Part model, mm, in its own coordinate system. A direction names the side the tool comes from. Give positions to 0.01 mm unless a question says otherwise; leave off trailing zeros. Write each loop counter-clockwise with the first axis right and the second up, starting at its lowest first coordinate (ties: lowest second). Pieces come first, ordered by that corner, then holes. Notation, with made-up numbers: M 26,28.25 L 52,28.25 A22 cw 52,44.25 Z; hole C -28,-16 d2. An arc over 180 degrees is marked long. Use a Markdown table: item, result.
```python
from build123d import *

# Parameters (mm, degrees)
F1_DEPTH = 4
F2_R     = 2.125
F3_DEPTH = 5.001
F4_W     = 8
F4_H     = 8
F5_DEPTH = 4
F6_R     = 2.125
F7_DEPTH = 22.001
F9_DEPTH = 4


with BuildPart() as f1:
    # F0 (on Top) → F1 (new body, symmetric)
    with BuildSketch(Plane.XY):
        with BuildLine():
            ThreePointArc((-3.2, -2.642442), (0, 4.15), (3.2, -2.642442))
            Line((3.2, -2.642442), (3.2, -17.642442))
            Line((3.2, -17.642442), (7, -17.642442))
            Line((7, -17.642442), (7, 2.35))
            Line((7, 2.35), (15, 2.35))
            Line((15, 2.35), (15, 7.35))
            Line((15, 7.35), (-15, 7.35))
            Line((-15, 7.35), (-15, 2.35))
            Line((-15, 2.35), (-7, 2.35))
            Line((-7, 2.35), (-7, -17.642442))
            Line((-7, -17.642442), (-3.2, -17.642442))
            Line((-3.2, -17.642442), (-3.2, -2.642442))
        make_face()
    extrude(amount=F1_DEPTH, both=True)

    # F2 (on face) → F3 (cut, through all)
    with BuildSketch(Plane.XZ.offset(-2.35)):
        with Locations((10, 0)):
            Circle(F2_R)
        with Locations((-10, 0)):
            Circle(F2_R)
    extrude(amount=-F3_DEPTH, mode=Mode.SUBTRACT)

    # F4 (on face) → F5 (join)
    with BuildSketch(Plane.XZ.offset(-2.35)):
        with Locations((11, 0)):
            Rectangle(F4_W, F4_H)
        Polygon((10, 3.377499), (12.925, 1.68875), (12.925, -1.68875), (10, -3.377499), (7.075, -1.68875), (7.075, 1.68875), align=None, mode=Mode.SUBTRACT)
        with Locations((-11, 0)):
            Rectangle(F4_W, F4_H)
        Polygon((-7.075, 1.68875), (-7.075, -1.68875), (-10, -3.377499), (-12.925, -1.68875), (-12.925, 1.68875), (-10, 3.377499), align=None, mode=Mode.SUBTRACT)
    extrude(amount=F5_DEPTH)

    # F6 (on face) → F7 (cut, through all)
    with BuildSketch(Plane.YZ.offset(7)):
        with Locations((-12.642442, 0)):
            Circle(F6_R)
    extrude(amount=-F7_DEPTH, mode=Mode.SUBTRACT)

    # F8 (on face) → F9 (join)
    with BuildSketch(Plane.YZ.offset(7)):
        Polygon((-14.951843, -4), (-10.333041, -4), (-8.02364, 0), (-10.333041, 4), (-14.951843, 4), (-17.261244, 0), align=None)
        Polygon((-12.642442, 3.377499), (-9.717442, 1.68875), (-9.717442, -1.68875), (-12.642442, -3.377499), (-15.567442, -1.68875), (-15.567442, 1.68875), align=None, mode=Mode.SUBTRACT)
    extrude(amount=F9_DEPTH)


solid = f1.part
```
1. Drop flat-ended pins along their axis: P1, Ø3, axis at y = -13, z = -2, coming from the +X side; P2, Ø1.5, axis at y = -10, z = -1, coming from the -X side; P3, Ø4, axis at x = 10, z = 0, coming from the +Y side. Give the stop position or say it passes through.
Findings below:
| item | result |
|---|---|
| P1 | x = 11 |
| P2 | x = -7 |
| P3 | y = -8.02 |
2. Cut at B-B, the plane y = -5.5. Give the cut face in (x, z).
Findings below:
| item | result |
|---|---|
| outline | M -7,-4 L -3.2,-4 L -3.2,4 L -7,4 Z; M 3.2,-4 L 7,-4 L 7,4 L 3.2,4 Z |
3. Drill centre lines: L1, parallel to X at y = 0, z = 0.5 (3 decimals); L2, parallel to X at y = -14.75, z = -3; L3, parallel to X at y = -3, z = 3.5. Where is each one in solid material? Low to high.
Findings below:
| item | result |
|---|---|
| L1 | -15 to -12.925, -7.075 to -4.15, 4.15 to 7.075, 12.925 to 15 |
| L2 | -7 to -3.2, 3.2 to 11 |
| L3 | -7 to -3.2, 3.2 to 7 |
4. Cut at D-D, the plane y = -12. Give the cut face in (x, z).
Findings below:
| item | result |
|---|---|
| outline | M -7,-4 L -3.2,-4 L -3.2,-2.03 L -7,-2.03 Z; M -7,2.03 L -3.2,2.03 L -3.2,4 L -7,4 Z; M 3.2,-4 L 11,-4 L 11,-3.01 L 7,-3.01 L 7,-2.03 L 3.2,-2.03 Z; M 3.2,2.03 L 7,2.03 L 7,3.01 L 11,3.01 L 11,4 L 3.2,4 Z |
5. Cut at A-A, the plane y = 0. State how many separate pieces and enclosed holes the cut face has, then the cut area to 3 significant figures.
Findings below:
| item | result |
|---|---|
| separate pieces | 2 |
| enclosed holes | 2 |
| area | 114 mm2 |
6. Tool access for faces 1 (the flat face through (8.97, -9.16, 1.97)), 2 (the flat face through (8.517, 0.378, 2.521)), 3 (the flat face through (-7.075, 0, 0)): list every direction of +Z, -Z, +X, -X, +Y, -Y with a clear straight run to the whole face (end or side of a thin tool).
Findings below:
| item | result |
|---|---|
| face 1 | +Z, +X |
| face 2 | none |
| face 3 | -Y |
7. Two-plate mould, pull along X, no slides. Class faces 4 (the flat face through (7, -13.3, -2.2)), 5 (the flat face through (8.972, -14.084, -2.545)), 6 (the flat face through (-12.925, 0, 0)): released by +X, released by -X, zero draft, split by the parting line, or undercut.
Findings below:
| item | result |
|---|---|
| face 4 | released by +X |
| face 5 | zero draft |
| face 6 | undercut |
